Part model, mm, in its own coordinate system. A direction names the side the tool comes from. Round coordinates to 2 decimals unless told otherwise and drop trailing zeros. Write each loop counter-clockwise with the first axis right and the second up, starting at its lowest first coordinate (ties: lowest second). Pieces come first, ordered by that corner, then holes.
1) Which spindle directions (+Z, -Z, +X, -X, +Y, -Y) get a long thin tool onto all of the face, cutting with end or side? Do faces 4 (the flat face through (30, 0, 2)), 5 (the cylindrical face through (40, 0, 33)), 6 (the flat face through (-30, 0, 32)). Say none if no direction does.
2) Pull direction Z, two halves, no side cores. Call faces 1 (the flat face through (20, 0, 17)), 2 (the flat face through (80, 0, -7.5)), 3 (the flat face through (15, -5, 6)): +Z half, -Z half, draft (parallel to the pull), parting line (faces both ways), or undercut.
3) Flat gauge pins, fed straight in: pin 1 (5 mm diameter, centred on y = 0, z = 20.5, fed in from +X); pin 2 (5 mm diameter, centred on x = 84.5, y = -1.5, fed in from +Z); pin 3 (6 mm diameter, centred on y = -2, z = -2.5, fed in from +X); pin 4 (3 mm diameter, centred on x = -35, y = 0, fed in from +Z). Where does each tip first touch, or does it go through?
4) Drill centre lines: L1, parallel to X at y = 0, z = 32.95; L2, parallel to X at y = 0, z = -9.5; L3, parallel to Z at x = 35.5, y = -3.5. Where is each one in solid material? Low to high.
5) Saw through at C-C on z = 18.5. Write the cut outline in (x, y).
6) Saw through at B-B on y = -3. Write the cut outline in (x, z).
7) Saw through at D-D on x = 96. Write the cut outline in (y, z).
8) Saw through at A-A on x = 23.5. Write the cut outline in (y, z), and give its area (3 significant figures).
```python
from build123d import *

# Parameters (mm, degrees)
EXTRUDE_1_DEPTH          = 34
SKETCH_2_R               = 1
CUT_EXTRUDE_4_DEPTH      = 35
CUT_EXTRUDE_4_DEPTH_BACK = 30
SKETCH_3_W               = 20
SKETCH_3_H               = 30
CUT_EXTRUDE_5_DEPTH      = 30
CUT_EXTRUDE_5_DEPTH_BACK = 30
EXTRUDE_4_DEPTH          = 15
SKETCH_5_R               = 1
CUT_EXTRUDE_7_DEPTH      = 16
SKETCH_6_W               = 15
SKETCH_6_H               = 10
EXTRUDE_5_DEPTH          = 10
SKETCH_7_W               = 70
SKETCH_7_H               = 10
CUT_EXTRUDE_8_DEPTH      = 10
CUT_EXTRUDE_8_DEPTH_BACK = 10


with BuildPart() as part:
    # 草圖1 → 填料-伸長1 (new body)
    with BuildSketch(Plane.XY):
        with BuildLine():
            Line((-35, 5), (35, 5))
            ThreePointArc((35, 5), (40, 0), (35, -5))
            Line((35, -5), (-35, -5))
            ThreePointArc((-35, -5), (-40, 0), (-35, 5))
        make_face()
    extrude(amount=EXTRUDE_1_DEPTH)

    # 草圖2 → 除料-伸長4 (cut, two sides)
    with BuildSketch(Plane.XY) as cut_extrude_4_sk:
        with Locations((-35, 0)):
            Circle(SKETCH_2_R)
        with Locations((35, 0)):
            Circle(SKETCH_2_R)
    extrude(amount=CUT_EXTRUDE_4_DEPTH, mode=Mode.SUBTRACT)
    extrude(cut_extrude_4_sk.sketch, amount=-CUT_EXTRUDE_4_DEPTH_BACK, mode=Mode.SUBTRACT)

    # 草圖3 → 除料-伸長5 (cut, two sides)
    with BuildSketch(Plane(origin=(0, 0, 0), x_dir=(1, 0, 0), z_dir=(0, 1, 0))) as cut_extrude_5_sk:
        with Locations((-30, -17)):
            Rectangle(SKETCH_3_W, SKETCH_3_H)
        with Locations((30, -17)):
            Rectangle(SKETCH_3_W, SKETCH_3_H)
    extrude(amount=CUT_EXTRUDE_5_DEPTH, mode=Mode.SUBTRACT)
    extrude(cut_extrude_5_sk.sketch, amount=-CUT_EXTRUDE_5_DEPTH_BACK, mode=Mode.SUBTRACT)

    # 草圖4 → 填料-伸長4 (add)
    with BuildSketch(Plane.XY):
        with BuildLine():
            Line((0, 5), (105, 5))
            ThreePointArc((105, 5), (110, 0), (105, -5))
            Line((105, -5), (0, -5))
            Line((0, -5), (0, 5))
        make_face()
    extrude(amount=-EXTRUDE_4_DEPTH)

    # 草圖5 → 除料-伸長7 (cut, through all)
    with BuildSketch(Plane.XY):
        with Locations((35, 0)):
            Circle(SKETCH_5_R)
        with Locations((105, 0)):
            Circle(SKETCH_5_R)
    extrude(amount=-CUT_EXTRUDE_7_DEPTH, mode=Mode.SUBTRACT)

    # 草圖6 → 填料-伸長5 (add)
    with BuildSketch(Plane(origin=(0, 0, 0), x_dir=(0, 0, -1), z_dir=(1, 0, 0))):
        with Locations((7.5, 0)):
            Rectangle(SKETCH_6_W, SKETCH_6_H)
    extrude(amount=-EXTRUDE_5_DEPTH)

    # 草圖7 → 除料-伸長8 (cut, two sides)
    with BuildSketch(Plane(origin=(0, 0, 0), x_dir=(1, 0, 0), z_dir=(0, 1, 0))) as cut_extrude_8_sk:
        with Locations((85, 2.5)):
            Rectangle(SKETCH_7_W, SKETCH_7_H)
    extrude(amount=CUT_EXTRUDE_8_DEPTH, mode=Mode.SUBTRACT)
    extrude(cut_extrude_8_sk.sketch, amount=-CUT_EXTRUDE_8_DEPTH_BACK, mode=Mode.SUBTRACT)


solid = part.part
```
Completed:
1. face 4: +X, +Y, -Y
1. face 5: +Z, +X
1. face 6: -X, +Y, -Y
2. face 1: undercut
2. face 2: +Z half
2. face 3: draft
3. pin 1: stops at x = 20
3. pin 2: stops at z = -7.5
3. pin 3: stops at x = 50
3. pin 4: stops at z = 34
4. L1: x = -40 to -36, -34 to 34, 36 to 40
4. L2: x = -10 to 34, 36 to 104, 106 to 110
4. L3: z = -15 to 2, 32 to 34
5. outline: (-20, -5) - (20, -5) - (20, 5) - (-20, 5) - close
6. outline: (-39, 0) - (-10, 0) - (-10, -15) - (109, -15) - (109, -7.5) - (50, -7.5) - (50, 0) - (39, 0) - (39, 2) - (20, 2) - (20, 32) - (39, 32) - (39, 34) - (-39, 34) - (-39, 32) - (-20, 32) - (-20, 2) - (-39, 2) - close
7. outline: (-5, -15) - (5, -15) - (5, -7.5) - (-5, -7.5) - close
8. outline: (-5, -15) - (5, -15) - (5, 2) - (-5, 2) - close; (-5, 32) - (5, 32) - (5, 34) - (-5, 34) - close
8. area: 190 mm2
